Could you check a few things on this model? Use its own coordinates, in mm. A direction names the side the tool comes from. Give positions to 0.01 mm unless a question says otherwise; leave off trailing zeros. Loops run counter-clockwise (first coordinate to the right, second up) from the corner with the lowest first, then second, coordinate; pieces in that order, holes last. Notation, with made-up numbers: (80, -31) - (131, -31) arc R30 ccw to (131, 6) - close; hole circle Ø6 at (35.5, 0.25). An arc over 180 degrees is marked (long way). One line per item, written item: value. Start each with the question number.
Q1. I want a section at A-A (z = -1.5). Please give me the cut outline in (x, y).
Q2. If we mould it in two halves opening along Y, with no side actions, what happens to faces 6 (the face through (-33, -6.629, 5)), 7 (the face through (-35.6, -13, 12)), 8 (the face through (-33, -20.069, 5)), 9 (the face through (-18, -28.08, 4))? For each: released by +Y, released by -Y, zero draft, split by the parting line, or undercut.
Q3. I'm going to push flat-ended pins straight in: P1, Ø1.5, axis at x = -34, y = -2, coming from the -Z side; P2, Ø6.5, axis at x = -8.5, y = -24.5, coming from the -Z side; P3, Ø3, axis at x = -28, y = -2.5, coming from the -Z side. Where does each tip first touch, or does it pass through?
Q4. If I drill on line 1 (Y direction, x = -33.1, z = 9.75); line 2 (Y direction, x = -2.6, z = 6); line 3 (Y direction, x = -22.5, z = 10), over which ranges is the centre line in solid material (lowest first)? Write a range as from..to.
Q5. For faces 1 (the face through (-18, 1, 12.92)), 2 (the face through (-8.1, -3, 11.9)), 3 (the face through (-2.6, -1.5, 0)), 4 (the face through (-18, -26.08, 4)), 5 (the face through (-18, -27, -4.2)), which set-ups out of +Z, -Z, +X, -X, +Y, -Y let a thin tool reach every point of the face, with its end or its side?
Q6. I want a section at B-B (x = -6.5). Please give me the cut outline in (y, z), then the cut area to 3 significant figures.
Q7. I want a section at C-C (z = 3.75). Please give me the cut outline in (x, y).
Q8. I want a section at D-D (x = -2.6). Please give me the cut outline in (y, z), then the cut area to 3 significant figures.
Autodesk Inventor part; units mm, degrees
ref_plane "Work Plane1" through (0, 0, 0) normal (0, 0, 1) x (1, 0, 0)
ref_plane "Work Plane2" through (-34.2906, -29.9214, 10.92) normal (0, 0, 1) x (0.9132, 0.4074, 0)
ref_plane "Work Plane3" through (-53.6, -42.75, -4.2) normal (0, 0, -1) x (0, 1, 0)
ref_plane "Work Plane1" through (0, 0, 0) normal (0, 0, 1) x (1, 0, 0)
sketch "Sketch1" plane through (0, 0, 0) normal (0, 0, 1) x (1, 0, 0)
  line L0 (0, -26.08) -> (0, 0)
  line L1 (0, 0) -> (-35.6, 0)
  line L2 (-35.6, -26.08) -> (0, -26.08)
  line L3 (-35.6, 0) -> (-35.6, -26.08)
  circle A0 centre (-2.6, -23.48) radius 1.45
  circle A1 centre (-2.6, -3.14) radius 1.45
  circle A2 centre (-33.1, -3.1792) radius 1.45
  circle A3 centre (-33.1, -23.5192) radius 1.45
  line L4 (-30.5, -20.0692) -> (-35.6, -20.0692)
  line L5 (-30.5, -6.6292) -> (-35.6, -6.6292)
  line L6 (-5.1, -5.6288) -> (0, -5.6288)
  line L7 (0, -5.6288) -> (0, 0)
  line L8 (-35.6, -26.08) -> (-35.6, -20.0692)
  line L9 (-35.6, -6.6292) -> (-35.6, 0)
  line L10 (0, -26.08) -> (0, -22.0692)
  line L11 (0, -22.0692) -> (0, -20.0692)
  line L12 (0, -20.0692) -> (-3.1, -20.0692)
  line L13 (-3.1, -20.0692) -> (-5.1, -20.0692)
  line L14 (-17.8, -25.74) -> (-5.1, -25.74)
  line L15 (-5.1, -25.74) -> (-5.1, -0.34)
  line L16 (-5.1, -0.34) -> (-30.5, -0.34)
  line L17 (-30.5, -0.34) -> (-30.5, -25.74)
  line L18 (-30.5, -25.74) -> (-17.8, -25.74)
  line L19 (-5.1, -25.74) -> (-5.1, -26.08)
  line L20 (-5.1, -26.08) -> (0, -26.08)
  line L21 (-30.5, -25.74) -> (-30.5, -26.08)
  line L22 (-35.6, -26.08) -> (-30.5, -26.08)
  line L23 (-30.5, -0.34) -> (-30.5, 0)
  line L24 (-30.5, 0) -> (-35.6, 0)
  line L25 (-5.1, -0.34) -> (-5.1, 0)
  line L26 (-5.1, 0) -> (0, 0)
  line L27 (-5.1, -26.08) -> (-30.5, -26.08)
  line L28 (-30.5, 0) -> (-5.1, 0)
  point P0 (-30.5, 0)
  point P1 (-5.1, 0)
ref_plane "Work Plane2" through (-34.2906, -29.9214, 10.92) normal (0, 0, 1) x (0.9132, 0.4074, 0)
extrude "Extrusion1" add sketch "Sketch1" along normal up to surface (10.92 mm away) contours L2 L19 L15 L13 L12 L0 | L2 L3 L4 L17 L21 | L6 L15 L25 L1 L0 | L3 L1 L23 L17 L5
sketch "Sketch2" plane through (-5.1, -26.08, 10.92) normal (0, 0, 1) x (1, 0, 0)
  line L0 (-30.5, 0) -> (5.1, 0)
  line L1 (5.1, 0) -> (5.1, 26.08)
  line L2 (0, 26.08) -> (5.1, 26.08)
  line L3 (5.1, 26.08) -> (-30.5, 26.08)
  line L4 (-30.5, 26.08) -> (-30.5, 0)
  circle A0 centre (-28, 2.5608) radius 1.45
  circle A1 centre (-28, 22.9008) radius 1.45
  circle A2 centre (2.5, 2.6) radius 1.45
  circle A3 centre (2.5, 22.94) radius 1.45
  line L5 (5.1, 0) -> (5.1, -2)
  line L6 (5.1, -2) -> (-30.5, -2)
  line L7 (-30.5, 0) -> (-25.4, 0)
  line L8 (-30.5, -2) -> (-30.5, 0)
  line L9 (-30.5, 19.4508) -> (-30.5, 26.08)
  line L10 (-30.5, 0) -> (-30.5, 26.08)
  line L11 (-30.5, 26.08) -> (-30.5, 28.08)
  line L12 (-30.5, 28.08) -> (0, 28.08)
  line L13 (0, 28.08) -> (5.1, 28.08)
  line L14 (5.1, 26.08) -> (5.1, 20.4512)
  line L15 (5.1, 28.08) -> (5.1, 26.08)
  line L16 (0, 20.4512) -> (0, 26.08)
  line L17 (0, 26.08) -> (0, 20.08)
  line L18 (0, 26.08) -> (-6, 26.08)
  line L19 (-6, 26.08) -> (0, 20.08)
  line L20 (-25.4, 19.4508) -> (-25.4, 26.08)
  line L21 (-25.4, 26.08) -> (-19.4, 26.08)
  line L22 (-25.4, 26.08) -> (-25.4, 20.08)
  line L23 (-25.4, 20.08) -> (-19.4, 26.08)
  line L24 (-25.4, 0) -> (-19.4, 0)
  line L25 (-25.4, 0) -> (-25.4, 6)
  line L26 (-25.4, 6.0108) -> (-25.4, 0)
  line L27 (-25.4, 6) -> (-19.4, 0)
  line L28 (0, 0) -> (-6, 0)
  line L29 (0, 6.0108) -> (0, 0)
  line L30 (0, 0) -> (0, 6)
  line L31 (0, 6) -> (-6, 0)
  line L32 (0, 6) -> (0, 20.08)
  line L33 (-25.4, 20.08) -> (-25.4, 6.0108)
  dimension "d19" = 2
  dimension "d20" = 2
  dimension "d21" = 6
  dimension "d22" = 6
  dimension "d23" = 6
  dimension "d24" = 6
  dimension "d25" = 6
  dimension "d26" = 6
  dimension "d27" = 6
  dimension "d28" = 6
extrude "Extrusion2" add sketch "Sketch2" along normal blind 2 contours L4 L3 L20 L33 L26 L25 L0 | L0 L5 L6 L8 | L25 L27 L0 | L11 L12 L13 L15 L2 L3 | L31 L29 L0 | L3 L23 L20 | L0 L29 L32 L17 L16 L2 L1 | L3 L16 L17 L19
ref_plane "Work Plane3" through (-53.6, -42.75, -4.2) normal (0, 0, -1) x (0, 1, 0)
extrude "Extrusion3" add sketch "Sketch2" against normal up to surface (15.12 mm away) contours L0 L5 L6 L8 | L11 L12 L13 L15 L2 L3
properties part number "gps_antenna_cover"
Worked answers:
1. outline: (-35.6, -28.08) - (0, -28.08) - (0, -26.08) - (-35.6, -26.08) - close; (-35.6, 0) - (0, 0) - (0, 2) - (-35.6, 2) - close
2. face 6: undercut
2. face 7: zero draft
2. face 8: undercut
2. face 9: released by -Y
3. P1: stops at z = 0
3. P2: stops at z = -4.2
3. P3: stops at z = 10.92
4. line 1: y = -28.08..-24.97, -22.07..-20.07, -6.63..-4.63, -1.73..2
4. line 2: y = -28.08..-24.93, -22.03..-20.07, -5.63..-4.59, -1.69..2
4. line 3: y = -28.08..-26.08, 0..2
5. face 1: +Z, +X, -X, +Y, -Y
5. face 2: +Z, -Z
5. face 3: -Z, +X, -X
5. face 4: -Z
5. face 5: -Z, +X, -X, +Y, -Y
6. outline: (-28.08, -4.2) - (-26.08, -4.2) - (-26.08, 10.92) - (-21.48, 10.92) - (-21.48, 12.92) - (-28.08, 12.92) - close; (-4.6, 10.92) - (0, 10.92) - (0, -4.2) - (2, -4.2) - (2, 12.92) - (-4.6, 12.92) - close
6. area: 86.9 mm²
7. outline: (-35.6, -28.08) - (0, -28.08) - (0, -20.07) - (-5.1, -20.07) - (-5.1, -26.08) - (-30.5, -26.08) - (-30.5, -20.07) - (-35.6, -20.07) - close; (-35.6, -6.63) - (-30.5, -6.63) - (-30.5, 0) - (-5.1, 0) - (-5.1, -5.63) - (0, -5.63) - (0, 2) - (-35.6, 2) - close; hole circle Ø2.9 at (-33.1, -23.52); hole circle Ø2.9 at (-33.1, -3.18); hole circle Ø2.9 at (-2.6, -23.48); hole circle Ø2.9 at (-2.6, -3.14)
8. outline: (-28.08, -4.2) - (-26.08, -4.2) - (-26.08, 0) - (-24.93, 0) - (-24.93, 12.92) - (-28.08, 12.92) - close; (-22.03, 0) - (-20.07, 0) - (-20.07, 10.92) - (-5.63, 10.92) - (-5.63, 0) - (-4.59, 0) - (-4.59, 12.92) - (-22.03, 12.92) - close; (-1.69, 0) - (0, 0) - (0, -4.2) - (2, -4.2) - (2, 12.92) - (-1.69, 12.92) - close
8. area: 173 mm²
